Geometry check sheet. Reference: the model listing, model coordinates, mm. Face numbers are marked on the shaded views. A direction names the side the tool comes from. Round coordinates to 2 decimals unless told otherwise and drop trailing zeros. Write each loop counter-clockwise with the first axis right and the second up, starting at its lowest first coordinate (ties: lowest second). Pieces come first, ordered by that corner, then holes.
Item 1: Access from +Z, -Z, +X, -X, +Y, -Y to the whole of each face (thin tool, end or side, straight path). Record for the marked faces 1 and 2.
Item 2: Depth check by flat-ended pin: P1, Ø3, axis at x = -16.5, z = 6, coming from the +Y side; P2, Ø5, axis at x = 20, y = 1, coming from the +Z side; P3, Ø5.5, axis at y = 35, z = 6.5, coming from the +X side; P4, Ø6, axis at x = -17.5, y = 28.5, coming from the -Z side. Enter the tip coordinate at first touch or a pass-through.
Item 3: Draft check along X on the marked faces 3 and 4. Enter one of: pulls with the +X half, pulls with the -X half, needs draft (parallel to the pull), parting line crosses it, or undercut.
Item 4: Cross-section at D-D (x = -33.5). Enter the section's corners in (y, z), then the cut area to 3 significant figures.
Item 5: Scan lines: probe 1 along Y at (x, z) = (50, 0.6); probe 2 along X at (y, z) = (35, 6.5); probe 3 along Y at (x, z) = (-17, 7.5). Record each from-to range of solid material in increasing order.
Item 6: Cross-section at C-C (z = 4.25). State how many separate pieces and enclosed holes the cut face has, then the cut area to 3 significant figures.
Item 7: Cross-section at B-B (x = -50). Enter the section's corners in (y, z), then the cut area to 3 significant figures.
Item 8: Cross-section at A-A (y = 34). Enter the section's corners in (x, z), then the cut area to 3 significant figures.
from build123d import *

# Parameters (mm, degrees)
SKETCH_1_W      = 108
SKETCH_1_H      = 76
SKETCH_1_R      = 1.5
EXTRUDE_1_DEPTH = 3
SKETCH_2_R      = 4
SKETCH_2_W      = 12
SKETCH_2_H      = 7
SKETCH_2_W_2    = 4
SKETCH_2_H_2    = 8
EXTRUDE_2_DEPTH = 8


with BuildPart() as part:
    # 草图1 → 凸台-拉伸1 (new body)
    with BuildSketch(Plane.XY):
        Rectangle(SKETCH_1_W, SKETCH_1_H)
        with Locations((-50, 34)):
            Circle(SKETCH_1_R, mode=Mode.SUBTRACT)
        with Locations((50, 34)):
            Circle(SKETCH_1_R, mode=Mode.SUBTRACT)
        with Locations((50, -34)):
            Circle(SKETCH_1_R, mode=Mode.SUBTRACT)
        with Locations((-50, -34)):
            Circle(SKETCH_1_R, mode=Mode.SUBTRACT)
    extrude(amount=EXTRUDE_1_DEPTH)

    # 草图2 → 凸台-拉伸2 (add)
    with BuildSketch(Plane.XY.offset(3)):
        with Locations((-27, 23)):
            Circle(SKETCH_2_R)
        with Locations((-7, 23)):
            Circle(SKETCH_2_R)
        with Locations((13, 23)):
            Circle(SKETCH_2_R)
        with Locations((33, 23)):
            Circle(SKETCH_2_R)
        with Locations(Location((33, -23, 0), (0, 0, 180))):
            Circle(SKETCH_2_R)
        with Locations(Location((13, -23, 0), (0, 0, 180))):
            Circle(SKETCH_2_R)
        with Locations(Location((-7, -23, 0), (0, 0, 180))):
            Circle(SKETCH_2_R)
        with Locations(Location((-27, -23, 0), (0, 0, 180))):
            Circle(SKETCH_2_R)
        with Locations((-33, 33.5)):
            Rectangle(SKETCH_2_W, SKETCH_2_H)
        with Locations((-13, 33.5)):
            Rectangle(SKETCH_2_W, SKETCH_2_H)
        with Locations((7, 33.5)):
            Rectangle(SKETCH_2_W, SKETCH_2_H)
        with Locations((27, 33.5)):
            Rectangle(SKETCH_2_W, SKETCH_2_H)
        with Locations((-37, 20)):
            Rectangle(SKETCH_2_W_2, SKETCH_2_H_2)
        with Locations((-17, 20)):
            Rectangle(SKETCH_2_W_2, SKETCH_2_H_2)
        with Locations((3, 20)):
            Rectangle(SKETCH_2_W_2, SKETCH_2_H_2)
        with Locations((23, 20)):
            Rectangle(SKETCH_2_W_2, SKETCH_2_H_2)
        with Locations((33, -33.5)):
            Rectangle(SKETCH_2_W, SKETCH_2_H)
        with Locations((13, -33.5)):
            Rectangle(SKETCH_2_W, SKETCH_2_H)
    extrude(amount=EXTRUDE_2_DEPTH)


solid = part.part
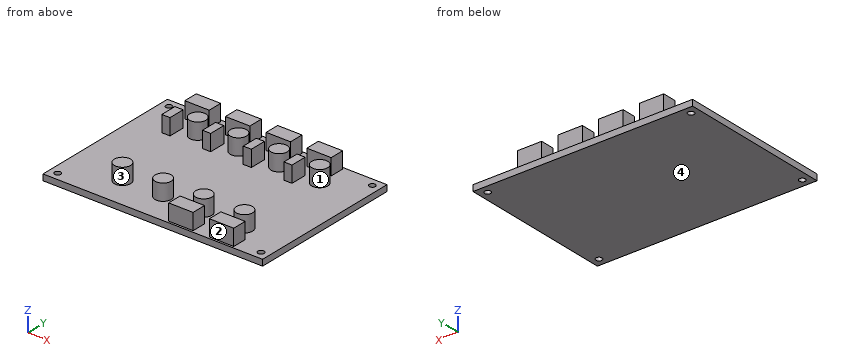
Resolved:
1. face 1: +Z
1. face 2: +Z, +X, -X, -Y
2. P1: stops at y = 37
2. P2: stops at z = 3
2. P3: stops at x = 33
2. P4: stops at z = 0
3. face 3: undercut
3. face 4: needs draft
4. outline: (-38, 0) - (38, 0) - (38, 3) - (37, 3) - (37, 11) - (30, 11) - (30, 3) - (-38, 3) - close
4. area: 284 mm2
5. probe 1: y = -38 to -35.5, -32.5 to 32.5, 35.5 to 38
5. probe 2: x = -39 to -27, -19 to -7, 1 to 13, 21 to 33
5. probe 3: y = 16 to 24, 30 to 37
6. separate pieces: 18
6. enclosed holes: 0
6. area: 1,030 mm2
7. outline: (-38, 0) - (-35.5, 0) - (-35.5, 3) - (-38, 3) - close; (-32.5, 0) - (32.5, 0) - (32.5, 3) - (-32.5, 3) - close; (35.5, 0) - (38, 0) - (38, 3) - (35.5, 3) - close
7. area: 210 mm2
8. outline: (-54, 0) - (-51.5, 0) - (-51.5, 3) - (-54, 3) - close; (-48.5, 0) - (48.5, 0) - (48.5, 3) - (33, 3) - (33, 11) - (21, 11) - (21, 3) - (13, 3) - (13, 11) - (1, 11) - (1, 3) - (-7, 3) - (-7, 11) - (-19, 11) - (-19, 3) - (-27, 3) - (-27, 11) - (-39, 11) - (-39, 3) - (-48.5, 3) - close; (51.5, 0) - (54, 0) - (54, 3) - (51.5, 3) - close
8. area: 690 mm2
